from build123d import *

# Parameters (mm, degrees)
SKETCH1_R           = 30
SKETCH1_R_2         = 1.6
BOSS_EXTRUDE1_DEPTH = 15
SKETCH2_R           = 20
CUT_EXTRUDE1_DEPTH  = 10
SKETCH3_R           = 18
BOSS_EXTRUDE2_DEPTH = 30
SKETCH4_R           = 16
CUT_EXTRUDE2_DEPTH  = 25
FILLET2_R           = 2


with BuildPart() as part:
    # Sketch1 → Boss-Extrude1 (new body)
    with BuildSketch(Plane.XY):
        Circle(SKETCH1_R)
        with Locations((-25, 0)):
            Circle(SKETCH1_R_2, mode=Mode.SUBTRACT)
        with Locations((25, 0)):
            Circle(SKETCH1_R_2, mode=Mode.SUBTRACT)
    extrude(amount=BOSS_EXTRUDE1_DEPTH)

    # Sketch2 → Cut-Extrude1 (cut)
    with BuildSketch(Plane.XY.offset(15)):
        Circle(SKETCH2_R)
    extrude(amount=-CUT_EXTRUDE1_DEPTH, mode=Mode.SUBTRACT)

    # Sketch3 → Boss-Extrude2 (add)
    with BuildSketch(Plane(origin=(0, 0, 0), x_dir=(-1, 0, 0), z_dir=(0, 0, -1))):
        Circle(SKETCH3_R)
    extrude(amount=BOSS_EXTRUDE2_DEPTH)

    # Sketch4 → Cut-Extrude2 (cut)
    with BuildSketch(Plane(origin=(0, 0, -30), x_dir=(-1, 0, 0), z_dir=(0, 0, -1))):
        Circle(SKETCH4_R)
    extrude(amount=-CUT_EXTRUDE2_DEPTH, mode=Mode.SUBTRACT)

    # Fillet2
    fillet2_edges = [part.edges().sort_by_distance(p)[0] for p in [
        (-30, 0, 0),
    ]]
    fillet(fillet2_edges, radius=FILLET2_R)


solid = part.part
Read the model definition and answer for the solid it produces. Units are mm, in the model's axes. A direction names the side the tool comes from. Coordinates: 2 decimals unless noted, no trailing zeros. Write each loop counter-clockwise with the first axis right and the second up, starting at its lowest first coordinate (ties: lowest second). Pieces come first, ordered by that corner, then holes. Notation, with made-up numbers: M 47,-21 L 57,-21 A23 cw 57,1 Z; hole C 66,-15 d11. An arc over 180 degrees is marked long. Use a Markdown table: item, result.
Q1. Which of the six approach directions +Z, -Z, +X, -X, +Y, -Y give full straight-line access (tool end or side, diameter ignored) to faces 1 (the face through (2.343, 17.847, -14.79)), 2 (the face through (-4.336, -19.524, 10.07)), 3 (the face through (12, -11, -30))?
Answer block:
| item | result |
|---|---|
| face 1 | -Z |
| face 2 | +Z |
| face 3 | -Z, +X, -X, +Y, -Y |
Q2. The part is cut by section A-A, the plane x = 0. Write down the section's boundary in (y, z), then the cut area to 3 significant figures.
Answer block:
| item | result |
|---|---|
| outline | M -30,2 A2 ccw -28,0 L -18,0 L -18,-30 L -16,-30 L -16,-5 L 16,-5 L 16,-30 L 18,-30 L 18,0 L 28,0 A2 ccw 30,2 L 30,15 L 20,15 L 20,5 L -20,5 L -20,15 L -30,15 Z |
| area | 778 mm2 |
Q3. The part is cut by section C-C, the plane z = -25. Write down the section's boundary in (x, y).
Answer block:
| item | result |
|---|---|
| outline | C 0,0 d36; hole C 0,0 d32 |
Q4. Each of these flat-tipped pins is pushed along its axis until it touches: pin 1 Ø8 at (y, z) = (8.5, -17.5) entering from -X; pin 2 Ø5 at (y, z) = (-5, 2) entering from -X; pin 3 Ø1 at (x, z) = (-16.5, -23) entering from +Y; pin 4 Ø1.9 at (x, y) = (-25, 0) entering from +Z. Where does it stop, or does it pass through?
Answer block:
| item | result |
|---|---|
| pin 1 | stops at x = -17.43 |
| pin 2 | stops at x = -29.9 |
| pin 3 | stops at y = 8.25 |
| pin 4 | passes through |
Q5. The part is cut by section D-D, the plane z = -4. Write down the section's boundary in (x, y), then the cut area to 3 significant figures.
Answer block:
| item | result |
|---|---|
| outline | C 0,0 d36 |
| area | 1,020 mm2 |
Q6. The part is cut by section B-B, the plane z = 10.5. Write down the section's boundary in (x, y), then the cut area to 3 significant figures.
Answer block:
| item | result |
|---|---|
| outline | C 0,0 d60; hole C -25,0 d3.2; hole C 0,0 d40; hole C 25,0 d3.2 |
| area | 1,550 mm2 |
Q7. Determine the mould class of faces 4 (the face through (6, -20, 15)), 5 (the face through (-29.97, 1.32, 8.41)), 6 (the face through (-26.18, 1.08, 7.4)) for opening direction Y: released by +Y, released by -Y, zero draft, split by the parting line, or undercut.
Answer block:
| item | result |
|---|---|
| face 4 | zero draft |
| face 5 | split by the parting line |
| face 6 | undercut |
Q8. Straight lines are drawn through the part: L1, parallel to Y at x = 0, z = -23.5; L2, parallel to Y at x = 0, z = 13; L3, parallel to Z at x = 20.5, y = 1.5. For each, find the intervals that lie inside material, in ascending order. Write a range as [from, to].
Answer block:
| item | result |
|---|---|
| L1 | y = [-18, -16], [16, 18] |
| L2 | y = [-30, -20], [20, 30] |
| L3 | z = [0, 15] |
